Print and shaded views of the part. All mm, measured from the part's lowest x, y and z. Round coordinates to 2 decimals unless told otherwise and drop trailing zeros. Write each loop counter-clockwise with the first axis right and the second up, starting at its lowest first coordinate (ties: lowest second). Pieces come first, ordered by that corner, then holes.
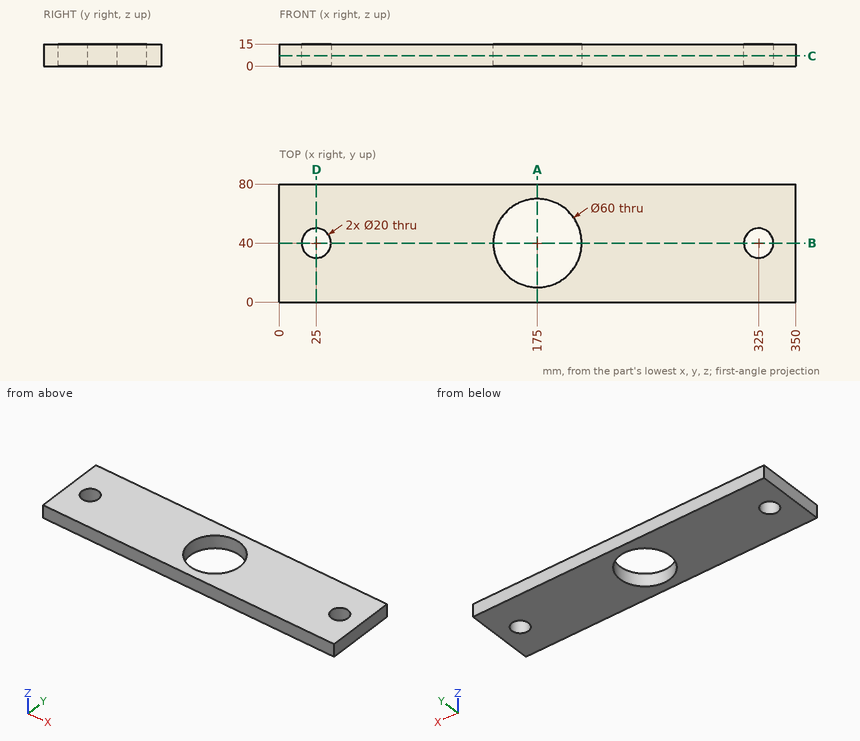
1) Wall check: L1, parallel to Y at x = 25, z = 11.5; L2, parallel to X at y = 44.5, z = 3.25; L3, parallel to Y at x = 175, z = 9.75. Give the ranges that are in metal, low to high.
Results:
L1: y = 0 to 30, 50 to 80
L2: x = 0 to 16.07, 33.93 to 145.34, 204.66 to 316.07, 333.93 to 350
L3: y = 0 to 10, 70 to 80
2) Slice it at D-D (x = 25). Write the cut outline in (y, z).
Results:
outline: (0, 0) - (30, 0) - (30, 15) - (0, 15) - close; (50, 0) - (80, 0) - (80, 15) - (50, 15) - close
3) Slice it at C-C (z = 7). Write the cut outline in (x, y), plus the area to 3 significant figures.
Results:
outline: (0, 0) - (350, 0) - (350, 80) - (0, 80) - close; hole circle Ø20 at (25, 40); hole circle Ø60 at (175, 40); hole circle Ø20 at (325, 40)
area: 24,500 mm2
4) Slice it at A-A (x = 175). Write the cut outline in (y, z), plus the area to 3 significant figures.
Results:
outline: (0, 0) - (10, 0) - (10, 15) - (0, 15) - close; (70, 0) - (80, 0) - (80, 15) - (70, 15) - close
area: 300 mm2
5) Slice it at B-B (y = 40). Write the cut outline in (x, z).
Results:
outline: (0, 0) - (15, 0) - (15, 15) - (0, 15) - close; (35, 0) - (145, 0) - (145, 15) - (35, 15) - close; (205, 0) - (315, 0) - (315, 15) - (205, 15) - close; (335, 0) - (350, 0) - (350, 15) - (335, 15) - close
